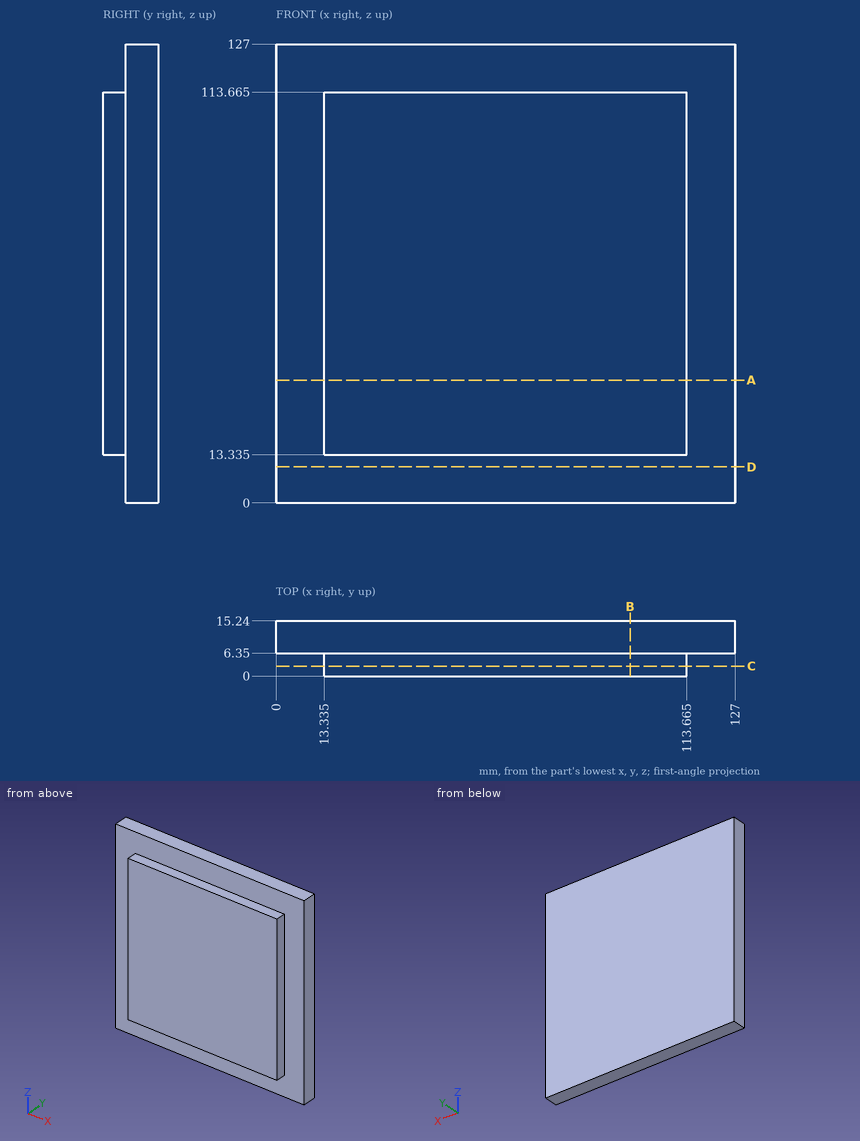
Input: dimensioned drawing with shaded views. Units: mm. Origin: part minimum x, y, z. Coordinates: 2 decimals unless noted, no trailing zeros. Loops run counter-clockwise (first coordinate to the right, second up) from the corner with the lowest first, then second, coordinate; pieces in that order, holes last. Notation, with made-up numbers: M 84.25,13 L 98.25,13 A14 cw 98.25,36 Z; hole C 40.5,26 d6. An arc over 180 degrees is marked long. One line per item, written item: value.
(1) Section D-D (z = 10). Output: boundary loops of the cut face in (x, y), and give its area (3 significant figures).
Filled in:
outline: M 0,6.35 L 127,6.35 L 127,15.24 L 0,15.24 Z
area: 1,130 mm^2
(2) Line query: line 1 along Z through (x, y) = (47, 3.5) (3 decimals); line 2 along Y through (x, z) = (5, 47). Output: solid intervals per line, ascending. Write a range as from..to.
Filled in:
line 1: 13.335..113.665
line 2: 6.35..15.24
(3) Section C-C (y = 2.75). Output: boundary loops of the cut face in (x, z) (3 decimals).
Filled in:
outline: M 13.335,13.335 L 113.665,13.335 L 113.665,113.665 L 13.335,113.665 Z
(4) Pin query (flat end, axial travel): pin 1 (2 mm diameter, centred on x = 106.5, z = 104.5, fed in from -Y); pin 2 (3 mm diameter, centred on y = 1.5, z = 45, fed in from +X) (3 decimals); pin 3 (3 mm diameter, centred on x = 76, y = 2, fed in from -Z) (3 decimals); pin 4 (3 mm diameter, centred on y = 2.5, z = 72, fed in from -X) (3 decimals). Return the tip coordinate at first contact, or that it passes through.
Filled in:
pin 1: y = 0
pin 2: x = 113.665
pin 3: z = 13.335
pin 4: x = 13.335
(5) Section B-B (x = 98). Output: boundary loops of the cut face in (y, z) (3 decimals), and give its area (3 significant figures).
Filled in:
outline: M 0,13.335 L 6.35,13.335 L 6.35,0 L 15.24,0 L 15.24,127 L 6.35,127 L 6.35,113.665 L 0,113.665 Z
area: 1,770 mm^2
(6) Section A-A (z = 34). Output: boundary loops of the cut face in (x, y) (3 decimals).
Filled in:
outline: M 0,6.35 L 13.335,6.35 L 13.335,0 L 113.665,0 L 113.665,6.35 L 127,6.35 L 127,15.24 L 0,15.24 Z
